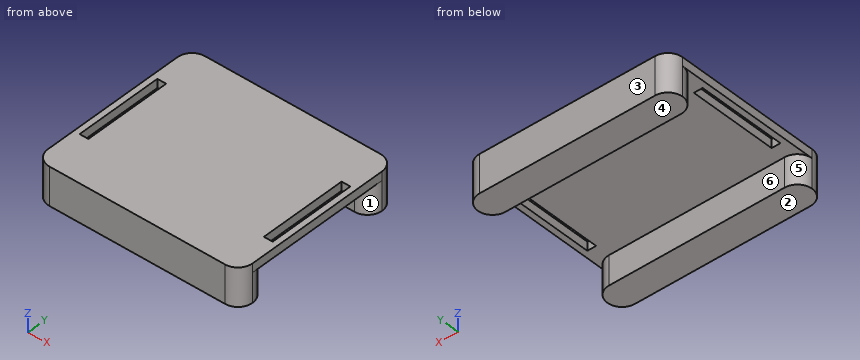
```python
from build123d import *

# Parameters (mm, degrees)
F0_W     = 70
F0_H     = 60
F1_DEPTH = 3
F2_W     = 3
F2_H     = 30
F3_DEPTH = 25
F4_W     = 70
F4_H     = 10
F5_DEPTH = 10
F6_R     = 4.99999


# Not quite as in the source:
# - a fillet or chamfer is up to 0.001 mm smaller than in the source, because OpenCascade refuses the exact size


with BuildPart() as f1:
    # F0 (on Top) → F1 (new body)
    with BuildSketch(Plane.XY):
        Rectangle(F0_W, F0_H)
    extrude(amount=F1_DEPTH)

    # F2 (on Top) → F3 (cut)
    with BuildSketch(Plane.XY):
        with Locations((31.5, 0)):
            Rectangle(F2_W, F2_H)
        with Locations((-31.5, 0)):
            Rectangle(F2_W, F2_H)
    extrude(amount=F3_DEPTH, mode=Mode.SUBTRACT)

    # F4 (on Top) → F5 (join)
    with BuildSketch(Plane.XY):
        with Locations((0, 25)):
            Rectangle(F4_W, F4_H)
        with Locations((0, -25)):
            Rectangle(F4_W, F4_H)
    extrude(amount=-F5_DEPTH)

    # F6 (radius 5 in the source; OpenCascade refuses exactly that, so slightly less here)
    f6_edges = [f1.edges().sort_by_distance(p)[0] for p in [
        (35, -30, -3.5),
        (-35, -30, -3.5),
        (-35, -20, -5),
        (35, -20, -5),
        (35, 20, -5),
        (35, 30, -3.5),
        (-35, 20, -5),
        (-35, 30, -3.5),
    ]]
    fillet(f6_edges, radius=F6_R)


solid = f1.part
```
Can you work these out from the model? Positions are in its coordinate system, mm. Face numbers are marked on the shaded views. A direction names the side the tool comes from. Coordinates: 2 decimals unless noted, no trailing zeros. Loops run counter-clockwise (first coordinate to the right, second up) from the corner with the lowest first, then second, coordinate; pieces in that order, holes last. Notation, with made-up numbers: M -27.75,20 L 15.25,20 A16 ccw 15.25,37 Z; hole C 35,4 d4. An arc over 180 degrees is marked long. Put each result on its own line as item: value. Start each with the question number.
(1) Imagine slicing it at A-A on y = -13. List the corners of the cut face in (x, z) for me.
(2) Will these pins go through, and if not, where does the flat tip stop? pin 1 Ø1 at (x, y) = (-8.5, 9) entering from -Z; pin 2 Ø3 at (y, z) = (22, -7.5) entering from +X; pin 3 Ø1.5 at (x, z) = (32, 2) entering from +Y.
(3) Imagine slicing it at D-D on z = 1.5. List the corners of the cut face in (x, y) for me, and give its area (3 significant figures).
(4) Which directions (+Z, -Z, +X, -X, +Y, -Y) give clear straight access to the entire face, cutting with the end or side of a thin tool? Please do the marked faces 1 and 2.
(5) I need wall thicknesses on probe 1 along X at (y, z) = (14, 1); probe 2 along Y at (x, z) = (29.5, -6.25); probe 3 along Z at (x, y) = (14.5, -12). Which ranges of each line are inside material? Lowest first, please.
(6) We'd pull the mould along Y, two halves only. Please class the marked faces 3, 4, 5 and 6: +Y half, -Y half, draft (parallel to the pull), parting line (faces both ways), or undercut.
(7) Imagine slicing it at C-C on x = -4. List the corners of the cut face in (y, z) for me.
Worked answers:
1. outline: M -35,0 L -33,0 L -33,3 L -35,3 Z; M -30,0 L 30,0 L 30,3 L -30,3 Z; M 33,0 L 35,0 L 35,3 L 33,3 Z
2. pin 1: stops at z = 0
2. pin 2: stops at x = 34.77
2. pin 3: stops at y = 29.84
3. outline: M -35,-25 A5 ccw -30,-30 L 30,-30 A5 ccw 35,-25 L 35,25 A5 ccw 30,30 L -30,30 A5 ccw -35,25 Z; hole M -33,-15 L -30,-15 L -30,15 L -33,15 Z; hole M 30,-15 L 33,-15 L 33,15 L 30,15 Z
3. area: 4,000 mm2
4. face 1: -Z, +X
4. face 2: -Z, +X, -X, +Y, -Y
5. probe 1: x = -35 to -33, -30 to 30, 33 to 35
5. probe 2: y = -30 to -20, 20 to 30
5. probe 3: z = 0 to 3
6. face 3: +Y half
6. face 4: draft
6. face 5: undercut
6. face 6: undercut
7. outline: M -30,-10 L -20,-10 L -20,0 L 20,0 L 20,-10 L 30,-10 L 30,3 L -30,3 Z
